Verification items for this drawing (mm, ordinates from the low corner). Round coordinates to 2 decimals unless told otherwise and drop trailing zeros. Order: outer loops, then holes, each group sorted by start corner. A loop starts at its lowest first (then second) coordinate and runs counter-clockwise, first axis right, second up. Notation, with made-up numbers: (-10.5, 43.25) -> (18.5, 43.25) arc R16 ccw to (18.5, 65.25) -> close; hole circle Ø10 at (59.25, 74.25). An arc over 180 degrees is marked (long way). Put each result on its own line as item: value.
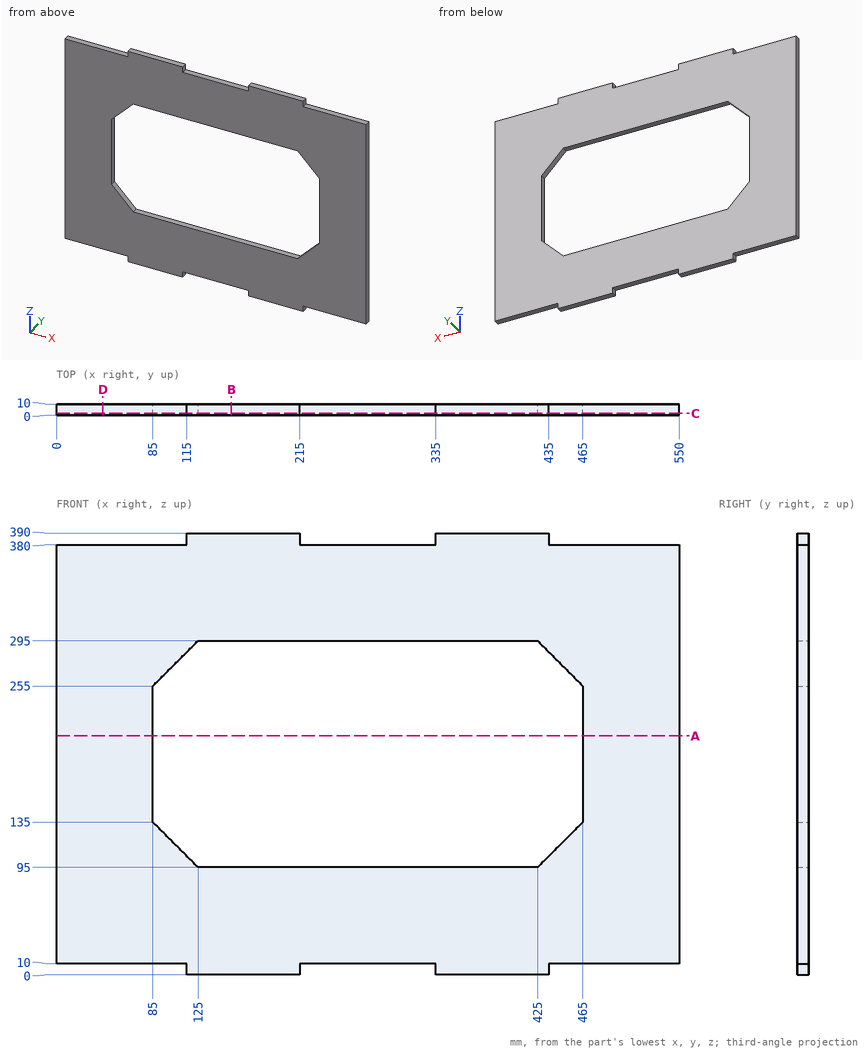
Item 1: Section check C-C on y = 1.75. Record the boundary of the cut face in (x, z), then the cut area to 3 significant figures.
Check sheet entries:
outline: (0, 10) -> (115, 10) -> (115, 0) -> (215, 0) -> (215, 10) -> (335, 10) -> (335, 0) -> (435, 0) -> (435, 10) -> (550, 10) -> (550, 380) -> (435, 380) -> (435, 390) -> (335, 390) -> (335, 380) -> (215, 380) -> (215, 390) -> (115, 390) -> (115, 380) -> (0, 380) -> close; hole (85, 135) -> (125, 95) -> (425, 95) -> (465, 135) -> (465, 255) -> (425, 295) -> (125, 295) -> (85, 255) -> close
area: 135,000 mm^2
Item 2: Section check A-A on z = 211. Record the boundary of the cut face in (x, y).
Check sheet entries:
outline: (0, 0) -> (85, 0) -> (85, 10) -> (0, 10) -> close; (465, 0) -> (550, 0) -> (550, 10) -> (465, 10) -> close
Item 3: Gauge pin test, flat ends, axial feed: pin 1 Ø5 at (x, y) = (261.5, 7) entering from -Z; pin 2 Ø5 at (y, z) = (6, 386) entering from +X; pin 3 Ø8 at (x, z) = (467, 247) entering from -Y; pin 4 Ø5 at (x, y) = (248, 2.5) entering from +Z. Record the tip position at first contact, or that the pin passes through.
Check sheet entries:
pin 1: stops at z = 10
pin 2: stops at x = 435
pin 3: stops at y = 0
pin 4: stops at z = 380
Item 4: Material ranges on L1, parallel to Z at x = 294.5, y = 5.25; L2, parallel to X at y = 5.5, z = 236.5; L3, parallel to Z at x = 171.5, y = 9, recorded low to high. Write a range as [from, to].
Check sheet entries:
L1: z = [10, 95], [295, 380]
L2: x = [0, 85], [465, 550]
L3: z = [0, 95], [295, 390]
Item 5: Section check B-B on x = 154.5. Record the boundary of the cut face in (y, z), then the cut area to 3 significant figures.
Check sheet entries:
outline: (0, 0) -> (10, 0) -> (10, 95) -> (0, 95) -> close; (0, 295) -> (10, 295) -> (10, 390) -> (0, 390) -> close
area: 1,900 mm^2
Item 6: Section check D-D on x = 41. Record the boundary of the cut face in (y, z).
Check sheet entries:
outline: (0, 10) -> (10, 10) -> (10, 380) -> (0, 380) -> close
